Read the model definition and answer for the solid it produces. Units are mm, in the model's axes. A direction names the side the tool comes from. Give positions to 0.01 mm unless a question says otherwise; leave off trailing zeros. Write each loop counter-clockwise with the first axis right and the second up, starting at its lowest first coordinate (ties: lowest second). Pieces come first, ordered by that corner, then holes.
```python
from build123d import *

# Parameters (mm, degrees)
F1_DEPTH      = 55
F1_DEPTH_BACK = 55
F2_R          = 2.5
F3_DEPTH      = 45.001
F5_DEPTH      = 55
F5_DEPTH_BACK = 55
F6_R          = 4.5
F7_DEPTH      = 6
F8_R          = 4.5
F9_DEPTH      = 6
F10_R         = 2
F11_DEPTH     = 3
F12_R         = 14
F13_DEPTH     = 3
F14_R         = 2.5
F15_DEPTH     = 3
F16_R         = 5
F17_DEPTH     = 3
F18_R         = 2
F19_DEPTH     = 3


with BuildPart() as f1:
    # F0 (on Top) → F1 (new body, two sides)
    with BuildSketch(Plane.XY) as f1_sk:
        with BuildLine():
            Line((-39, 45), (-42, 45))
            Line((-42, 45), (-42, -15))
            ThreePointArc((-42, -15), (-40.242641, -19.242641), (-36, -21))
            Line((-36, -21), (-6, -21))
            ThreePointArc((-6, -21), (-1.757359, -19.242641), (0, -15))
            ThreePointArc((0, -15), (1.757359, -19.242641), (6, -21))
            Line((6, -21), (19.753644, -21))
            Line((19.753644, -21), (19.753644, -18))
            Line((19.753644, -18), (6, -18))
            ThreePointArc((6, -18), (3.87868, -17.12132), (3, -15))
            Line((3, -15), (3, 0))
            Line((3, 0), (-3, 0))
            Line((-3, 0), (-3, -15))
            ThreePointArc((-3, -15), (-3.87868, -17.12132), (-6, -18))
            Line((-6, -18), (-36, -18))
            ThreePointArc((-36, -18), (-38.12132, -17.12132), (-39, -15))
            Line((-39, -15), (-39, 45))
        make_face()
    extrude(amount=F1_DEPTH)
    extrude(f1_sk.sketch, amount=-F1_DEPTH_BACK)

    # F2 (on face) → F3 (cut, through all)
    with BuildSketch(Plane.YZ.offset(3)):
        with Locations((-5, 45)):
            Circle(F2_R)
        with Locations((-5, 0)):
            Circle(F2_R)
        with Locations((-5, -45)):
            Circle(F2_R)
    extrude(amount=-F3_DEPTH, mode=Mode.SUBTRACT)

    # F4 (on Top) → F5 (join, two sides)
    with BuildSketch(Plane.XY) as f5_sk:
        with BuildLine():
            Line((-42, -15), (-42, 45))
            Line((-42, 45), (-45, 45))
            Line((-45, 45), (-45, -15))
            ThreePointArc((-45, -15), (-45.87868, -17.12132), (-48, -18))
            Line((-48, -18), (-164, -18))
            Line((-164, -18), (-164, -21))
            Line((-164, -21), (-48, -21))
            ThreePointArc((-48, -21), (-43.757359, -19.242641), (-42, -15))
        make_face()
    extrude(amount=F5_DEPTH)
    extrude(f5_sk.sketch, amount=-F5_DEPTH_BACK)

    # F6 (on face) → F7 (cut)
    with BuildSketch(Plane.YZ.offset(-39)):
        with Locations((-5, 45)):
            Circle(F6_R)
        with Locations((-5, 0)):
            Circle(F6_R)
        with Locations((-5, -45)):
            Circle(F6_R)
    extrude(amount=-F7_DEPTH, mode=Mode.SUBTRACT)

    # F8 (on face) → F9 (cut)
    with BuildSketch(Plane.YZ.offset(-39)):
        with Locations((37, 0)):
            Circle(F8_R)
        with Locations((37, -45)):
            Circle(F8_R)
        with Locations((37, 45)):
            Circle(F8_R)
    extrude(amount=-F9_DEPTH, mode=Mode.SUBTRACT)

    # F10 (on face) → F11 (cut)
    with BuildSketch(Plane.XZ.offset(21)):
        with Locations((-30.246356, -34)):
            Circle(F10_R)
        with Locations((-30.246356, 34)):
            Circle(F10_R)
        with Locations((-125.246356, 34)):
            Circle(F10_R)
        with Locations((-125.246356, -34)):
            Circle(F10_R)
    extrude(amount=-F11_DEPTH, mode=Mode.SUBTRACT)

    # F12 (on face) → F13 (cut)
    with BuildSketch(Plane.XZ.offset(21)):
        with Locations((-68.651619, -27.215034)):
            Circle(F12_R)
    extrude(amount=-F13_DEPTH, mode=Mode.SUBTRACT)

    # F14 (on face) → F15 (cut)
    with BuildSketch(Plane.XZ.offset(21)):
        with Locations((-159.7, 29.7)):
            Circle(F14_R)
        with Locations((-159.7, -30.3)):
            Circle(F14_R)
        with Locations((-77.7, 29.7)):
            Circle(F14_R)
        with Locations((-77.7, -45.3)):
            Circle(F14_R)
    extrude(amount=-F15_DEPTH, mode=Mode.SUBTRACT)

    # F16 (on face) → F17 (cut)
    with BuildSketch(Plane.XZ.offset(21)):
        with Locations((-112.746356, -26)):
            Circle(F16_R)
    extrude(amount=-F17_DEPTH, mode=Mode.SUBTRACT)

    # F18 (on face) → F19 (cut)
    with BuildSketch(Plane.XZ.offset(21)):
        with Locations((-76.393303, 13.251823)):
            Circle(F18_R)
        with Locations((-160.16324, -15.807402)):
            Circle(F18_R)
    extrude(amount=-F19_DEPTH, mode=Mode.SUBTRACT)


solid = f1.part
```
Item 1: Which of the six approach directions +Z, -Z, +X, -X, +Y, -Y give full straight-line access (tool end or side, diameter ignored) to faces 4 (the cylindrical face through (-41.96, -5.59, 4.46)), 5 (the flat face through (-45, 15, -1)), 6 (the cylindrical face through (-41.96, 39.08, 41.01))?
Result set:
face 4: -X
face 5: +Z, -Z, -X, +Y
face 6: +X, -X
Item 2: Section A-A (y = -5) is taken. Give the number of separate pieces and of enclosed holes in the cut face, and give its area (3 significant figures).
Result set:
separate pieces: 8
enclosed holes: 0
area: 1,070 mm2
Item 3: Find the intervals of material crossed by line 1 along Z through (x, y) = (1.4, -5); line 2 along X through (y, z) = (-6, -14); line 3 along X through (y, z) = (28.5, 18), in increasing order.
Result set:
line 1: z = -55 to -47.5, -42.5 to -2.5, 2.5 to 42.5, 47.5 to 55
line 2: x = -45 to -39, -3 to 3
line 3: x = -45 to -39
Item 4: Each of these flat-tipped pins is pushed along its axis until it touches: pin 1 Ø10.5 at (y, z) = (37, 45) entering from +X; pin 2 Ø5 at (x, y) = (-7.5, -0.5) entering from -Z; pin 3 Ø12 at (x, z) = (-25.5, 38.5) entering from +Y; pin 4 Ø6.5 at (y, z) = (-5, -45) entering from -X. Where does it stop, or does it pass through?
Result set:
pin 1: stops at x = -39
pin 2: passes through
pin 3: stops at y = -18
pin 4: stops at x = -3
Item 5: Section C-C (y = -13) is taken. Write down the section's boundary in (x, z).
Result set:
outline: (-45, -55) - (-39, -55) - (-39, 55) - (-45, 55) - close; (-3, -55) - (3, -55) - (3, 55) - (-3, 55) - close
Item 6: Determine the mould class of faces 1 (the flat face through (-3, -9, 1)), 2 (the cylindrical face through (0.042, -2.615, 0.751)), 3 (the flat face through (-105, -18, -1)) for opening direction Y: pulls with the +Y half, pulls with the -Y half, needs draft (parallel to the pull), parting line crosses it, or undercut.
Result set:
face 1: needs draft
face 2: undercut
face 3: pulls with the +Y half
